Could you check a few things on this drawing? It's one solid part, dimensions in mm from its lowest x, y, z. Coordinates: 2 decimals unless noted, no trailing zeros. Order: outer loops, then holes, each group sorted by start corner. A loop starts at its lowest first (then second) coordinate and runs counter-clockwise, first axis right, second up. Notation, with made-up numbers: (18.25, 71) - (31.25, 71) arc R19 cw to (31.25, 107) - close; hole circle Ø9 at (-15.5, 63). An arc over 180 degrees is marked (long way). Return JSON: item names as keys, results as strings. Group by question number.
1) Imagine slicing it at D-D (y = 12). Write out the boundary of the cut face in (x, z), and give its area (3 significant figures).
2) Imagine slicing it at A-A (y = 10). Write out the boundary of the cut face in (x, z), and give its area (3 significant figures).
3) If I drill on line 1 along Y through (x, z) = (27, 0.15); line 2 along X through (y, z) = (11.5, 0.25); line 3 along X through (y, z) = (11, 0.3), over which ranges is the centre line in solid material (lowest first)?
4) Imagine slicing it at B-B (x = 27). Write out the boundary of the cut face in (y, z).
5) Imagine slicing it at C-C (z = 0.4). Write out the boundary of the cut face in (x, y).
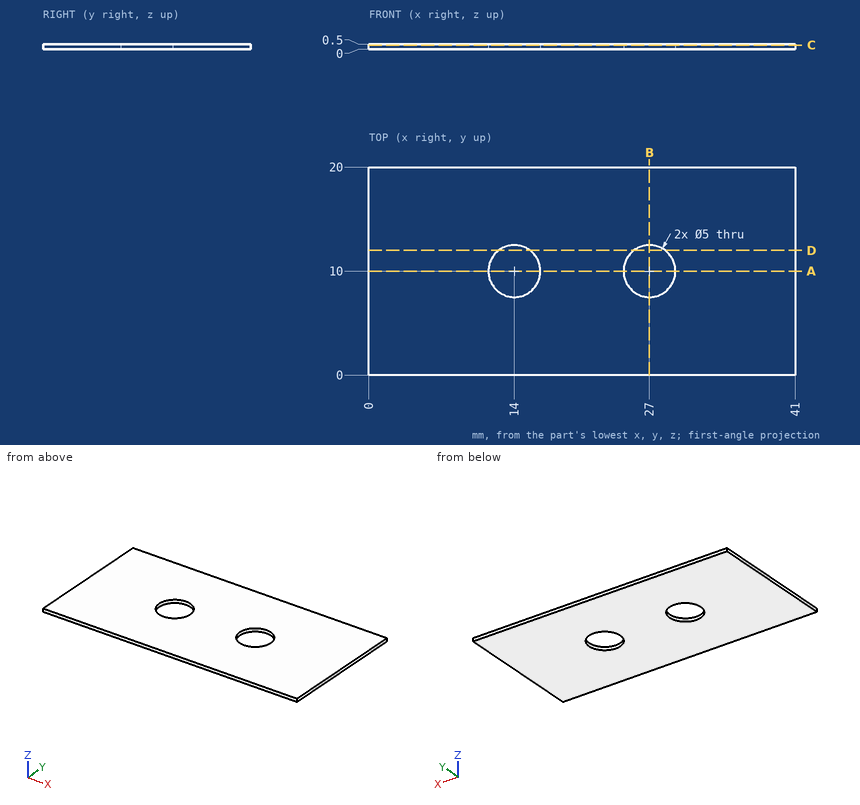
Calculated:
{
 "1": {"outline": "(0, 0) - (12.5, 0) - (12.5, 0.5) - (0, 0.5) - close; (15.5, 0) - (25.5, 0) - (25.5, 0.5) - (15.5, 0.5) - close; (28.5, 0) - (41, 0) - (41, 0.5) - (28.5, 0.5) - close", "area": "17.5 mm2"},
 "2": {"outline": "(0, 0) - (11.5, 0) - (11.5, 0.5) - (0, 0.5) - close; (16.5, 0) - (24.5, 0) - (24.5, 0.5) - (16.5, 0.5) - close; (29.5, 0) - (41, 0) - (41, 0.5) - (29.5, 0.5) - close", "area": "15.5 mm2"},
 "3": {"line 1": "0 to 7.5, 12.5 to 20", "line 2": "0 to 12, 16 to 25, 29 to 41", "line 3": "0 to 11.71, 16.29 to 24.71, 29.29 to 41"},
 "4": {"outline": "(0, 0) - (7.5, 0) - (7.5, 0.5) - (0, 0.5) - close; (12.5, 0) - (20, 0) - (20, 0.5) - (12.5, 0.5) - close"},
 "5": {"outline": "(0, 0) - (41, 0) - (41, 20) - (0, 20) - close; hole circle Ø5 at (14, 10); hole circle Ø5 at (27, 10)"}
}
